The figure shows three views and two pictorial views of one solid part (mm, origin at its lowest corner). Answer the questions. A direction names the side the tool comes from. Round coordinates to 2 decimals unless told otherwise and drop trailing zeros. Order: outer loops, then holes, each group sorted by start corner. A loop starts at its lowest first (then second) coordinate and runs counter-clockwise, first axis right, second up. Notation, with made-up numbers: (-14, 47.5) - (12, 47.5) arc R21 cw to (12, 61.5) - close; hole circle Ø3 at (-26.75, 87.25). An arc over 180 degrees is marked (long way). Answer as a JSON object with one key per item and string values. Group by question number.
Q1. Given pin 1 Ø2 at (x, y) = (128, 48) entering from +Z, flat-ended and moving along its own axis, determine where the tip first touches the part or whether it passes through.
Q2. A cutting plane is placed at B-B on y = 154. Determine the outline of the cut face in (x, z), and give its area (3 significant figures).
Q3. A cutting plane is placed at A-A on x = 125. Determine the outline of the cut face in (y, z), and give its area (3 significant figures).
Q4. The mould has two halves that part along Y. Classify the marked faces 1, 2 and 3: pulls with the +Y half, pulls with the -Y half, needs draft (parallel to the pull), parting line crosses it, or undercut.
Q5. A tool of negligible diameter and unlimited length cuts with its end or side. For the marked faces 4 and 5, from which of +Z, -Z, +X, -X, +Y, -Y can it reach the whole face along a straight path? Write none if from no direction.
Q6. A cutting plane is placed at C-C on z = 119. Determine the outline of the cut face in (x, y).
Q7. Consider line 1 (Y direction, x = 69, z = 63.5); line 2 (X direction, y = 82.5, z = 126); line 3 (Z direction, x = 107, y = 162). Determine where each line is inside the solid, lowest interval first.
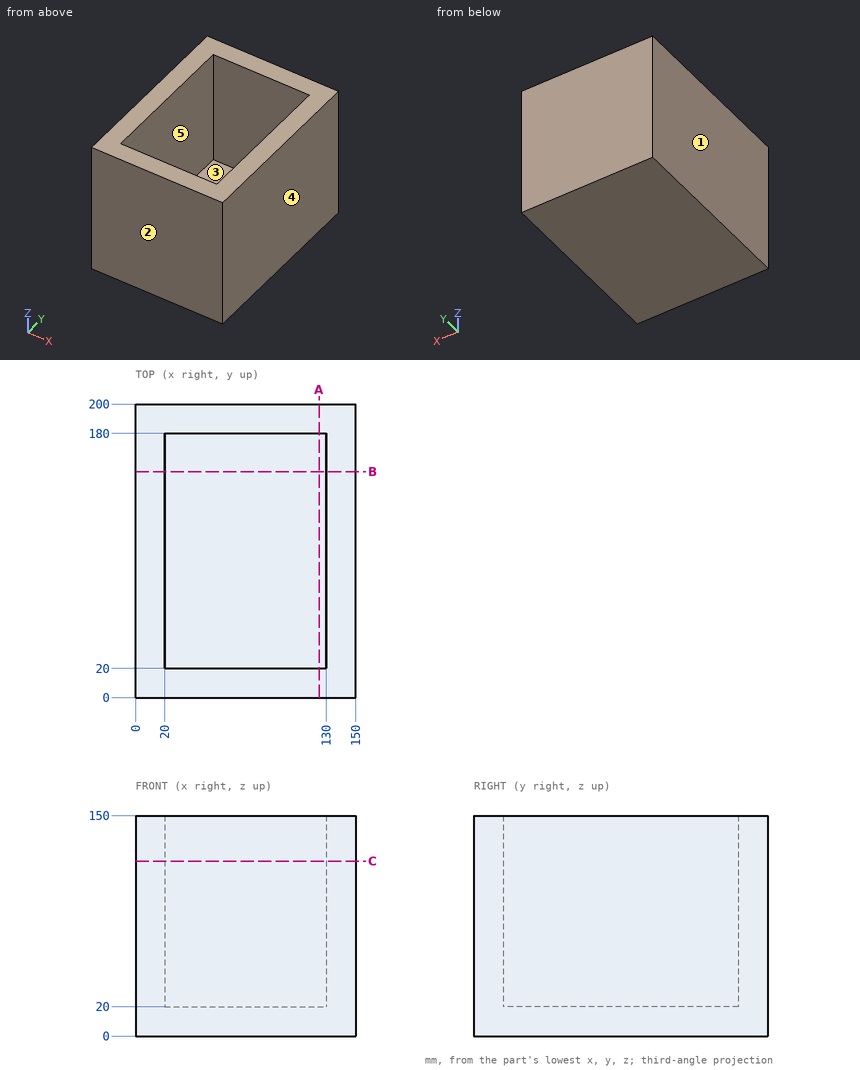
Result set:
{
 "1": {"pin 1": "stops at z = 20"},
 "2": {"outline": "(0, 0) - (150, 0) - (150, 150) - (130, 150) - (130, 20) - (20, 20) - (20, 150) - (0, 150) - close", "area": "8,200 mm²"},
 "3": {"outline": "(0, 0) - (200, 0) - (200, 150) - (180, 150) - (180, 20) - (20, 20) - (20, 150) - (0, 150) - close", "area": "9,200 mm²"},
 "4": {"face 1": "needs draft", "face 2": "pulls with the -Y half", "face 3": "undercut"},
 "5": {"face 4": "+Z, -Z, +X, +Y, -Y", "face 5": "+Z"},
 "6": {"outline": "(0, 0) - (150, 0) - (150, 200) - (0, 200) - close; hole (20, 20) - (130, 20) - (130, 180) - (20, 180) - close"},
 "7": {"line 1": "y = 0 to 20, 180 to 200", "line 2": "x = 0 to 20, 130 to 150", "line 3": "z = 0 to 20"}
}
